Could you check a few things on this model? Use its own coordinates, in mm. A direction names the side the tool comes from. Coordinates: 2 decimals unless noted, no trailing zeros. Order: outer loops, then holes, each group sorted by start corner. A loop starts at its lowest first (then second) coordinate and runs counter-clockwise, first axis right, second up. Notation, with made-up numbers: (38, -11) - (77, -11) arc R20 ccw to (77, -2) - close; hole circle Ø3 at (34.5, 42). An arc over 180 degrees is marked (long way). One line per item, written item: value. Start each with the question number.
from build123d import *

# Parameters (mm, degrees)
SKETCH1_W           = 56.55
SKETCH1_H           = 23.65
BOSS_EXTRUDE1_DEPTH = 20
CUT_EXTRUDE1_DEPTH  = 12


with BuildPart() as part:
    # Sketch1 → Boss-Extrude1 (new body)
    with BuildSketch(Plane.XY):
        Rectangle(SKETCH1_W, SKETCH1_H)
    extrude(amount=BOSS_EXTRUDE1_DEPTH)

    # Sketch2 → Cut-Extrude1 (cut)
    with BuildSketch(Plane.XY.offset(20)):
        with BuildLine():
            Line((-20.5, 5.825), (-17.5, 5.825))
            Line((-17.5, 5.825), (-14.5, 5.825))
            ThreePointArc((-14.5, 5.825), (-17.5, 8.825), (-20.5, 5.825))
        make_face()
        with BuildLine():
            Line((-14.5, 5.825), (-17.5, 5.825))
            Line((-17.5, 5.825), (-20.5, 5.825))
            ThreePointArc((-20.5, 5.825), (-17.5, 2.825), (-14.5, 5.825))
        make_face()
        with BuildLine():
            ThreePointArc((20.5, 5.825), (17.5, 8.825), (14.5, 5.825))
            Line((14.5, 5.825), (17.5, 5.825))
            Line((17.5, 5.825), (20.5, 5.825))
        make_face()
        with BuildLine():
            Line((17.5, 5.825), (14.5, 5.825))
            ThreePointArc((14.5, 5.825), (17.5, 2.825), (20.5, 5.825))
            Line((20.5, 5.825), (17.5, 5.825))
        make_face()
    extrude(amount=-CUT_EXTRUDE1_DEPTH, mode=Mode.SUBTRACT)


solid = part.part
Q1. We'd pull the mould along Y, two halves only. Please class faces 1 (the flat face through (0, -11.825, 10)), 2 (the cylindrical face through (-15.12, 7.65, 14.08)), 3 (the flat face through (0, 0, 0)), 4 (the flat face through (0, 11.825, 10)): +Y half, -Y half, draft (parallel to the pull), parting line (faces both ways), or undercut.
Q2. If I drill on L1, parallel to X at y = 6, z = 17.75 (3 decimals); L2, parallel to Y at x = 17.5, z = 14.25 (3 decimals); L3, parallel to X at y = 8.5, z = 8.5 (3 decimals), over which ranges is the centre line in solid material (lowest first)?
Q3. I want a section at C-C on y = 4.25. Please give me the cut outline in (x, z) (3 decimals), then the cut area to 3 significant figures.
Q4. I want a section at A-A on z = 12.5. Please give me the cut outline in (x, y) (3 decimals), then the cut area to 3 significant figures.
Q5. I want a section at B-B on x = 17.5. Please give me the cut outline in (y, z) (3 decimals), then the cut area to 3 significant figures.
Q6. Which directions (+Z, -Z, +X, -X, +Y, -Y) give clear straight access to the entire face, cutting with the end or side of a thin tool? Please do faces 5 (the flat face through (28.275, 0, 10)), 6 (the flat face through (-18, 6, 8)).
Values follow:
1. face 1: -Y half
1. face 2: undercut
1. face 3: draft
1. face 4: +Y half
2. L1: x = -28.275 to -20.495, -14.505 to 14.505, 20.495 to 28.275
2. L2: y = -11.825 to 2.825, 8.825 to 11.825
2. L3: x = -28.275 to -18.858, -16.142 to 16.142, 18.858 to 28.275
3. outline: (-28.275, 0) - (28.275, 0) - (28.275, 20) - (20.053, 20) - (20.053, 8) - (14.947, 8) - (14.947, 20) - (-14.947, 20) - (-14.947, 8) - (-20.053, 8) - (-20.053, 20) - (-28.275, 20) - close
3. area: 1,010 mm^2
4. outline: (-28.275, -11.825) - (28.275, -11.825) - (28.275, 11.825) - (-28.275, 11.825) - close; hole circle Ø6 at (-17.5, 5.825); hole circle Ø6 at (17.5, 5.825)
4. area: 1,280 mm^2
5. outline: (-11.825, 0) - (11.825, 0) - (11.825, 20) - (8.825, 20) - (8.825, 8) - (2.825, 8) - (2.825, 20) - (-11.825, 20) - close
5. area: 401 mm^2
6. face 5: +Z, -Z, +X, +Y, -Y
6. face 6: +Z
